Input: part model. Units: mm. Frame: model coordinates. Face numbers are marked on the shaded views. A direction names the side the tool comes from. Coordinates: 2 decimals unless noted, no trailing zeros. Write each loop counter-clockwise with the first axis right and the second up, starting at its lowest first coordinate (ties: lowest second). Pieces come first, ordered by that corner, then holes. Notation, with made-up numbers: (66, 16) - (118, 16) arc R34 ccw to (118, 55) - close; hole circle Ø3 at (85, 67.25). An arc over 180 degrees is marked (long way). Use a Markdown table: item, result. Add a question column.
Q1. Pin query (flat end, axial travel): P1, Ø8, axis at x = 9, y = -29, coming from the -Z side; P2, Ø3.5, axis at y = -22.225, z = 0, coming from the +X side; P3, Ø1, axis at x = 15.5, z = -0.5, coming from the +Y side; P4, Ø12, axis at y = -14.5, z = -1, coming from the +X side. Return the tip coordinate at first contact, or that it passes through.
Q2. Section query D-D (z = 0). Give the number of separate pieces and of enclosed holes in the cut face, then the cut area to 3 significant figures.
Q3. Section query A-A (z = -5.25). Return the cut outline in (x, y).
Q4. Section query B-B (y = -17). Return the cut outline in (x, z), then the cut area to 3 significant figures.
Q5. Section query C-C (x = 13.5). Return the cut outline in (y, z).
Q6. Set-up query: the marked faces 1 and 2. Return all of +Z, -Z, +X, -X, +Y, -Y with unobstructed straight access to the full face (end or side cutting, diameter ignored); none if empty.
Q7. Material intervals for probe 1 along Y at (x, z) = (0.55, 0); probe 2 along Y at (x, z) = (-0.3, 0); probe 3 along X at (y, z) = (-19.5, 10), sorted ascending. Write a range as from..to.
from build123d import *

# Parameters (mm, degrees)
SKETCH2_W                       = 3.175
SKETCH2_H                       = 25.4
F_1_8_0_125_DIAMETER_HOLE1_D    = 3.175
F_3_32_0_09375_DIAMETER_HOLE2_D = 2.38125
FILLET1_R                       = 12.7
FILLET2_R                       = 6.35
CHAMFER3_SIZE                   = 0.762
CHAMFER2_SIZE                   = 0.254


with BuildPart() as part:
    # Sweep1: sweep along a path in Sketch1
    with BuildLine(Plane.XY) as sweep1_path:
        Line((0, 0), (0, -31.75))
        Line((0, -31.75), (0, -70.0334134))
        Line((0, -70.0334134), (27.49630657, -85.9084134))
    # Sketch2 → Sweep1 (sweep)
    with BuildSketch(Plane(origin=(0, 0, 0), x_dir=(1, 0, 0), z_dir=(0, 1, 0))):
        Rectangle(SKETCH2_W, SKETCH2_H)
    sweep(path=sweep1_path.line, transition=Transition.RIGHT)

    # 1/8 (0.125) Diameter Hole1 (through all)
    with Locations(Plane(origin=(1.5875, 0, 0), x_dir=(0, 0, -1), z_dir=(1, 0, 0))):
        with Locations((0, -9.525), (0, -22.225)):
            Hole(F_1_8_0_125_DIAMETER_HOLE1_D / 2)

    # 3/32 (0.09375) Diameter Hole2 (through all)
    with Locations(Plane(origin=(-29.531607559, -51.150244721, 0), x_dir=(0.866025404, -0.5, 0), z_dir=(0.5, 0.866025404, 0))):
        with Locations((57.2417067, 0)):
            Hole(F_3_32_0_09375_DIAMETER_HOLE2_D / 2)

    # Fillet1
    fillet1_edges = [part.edges().sort_by_distance(p)[0] for p in [
        (1.5875, -69.116869848, 0),
        (-1.5875, -70.949956952, 0),
    ]]
    fillet(fillet1_edges, radius=FILLET1_R)

    # Fillet2
    fillet2_edges = [part.edges().sort_by_distance(p)[0] for p in [
        (27.49630657, -85.9084134, -12.7),
        (27.49630657, -85.9084134, 12.7),
        (0, 0, -12.7),
        (0, 0, 12.7),
    ]]
    fillet(fillet2_edges, radius=FILLET2_R)

    # Chamfer3
    chamfer3_edges = [part.edges().sort_by_distance(p)[0] for p in [
        (12.982897628, -79.362179945, -12.7),
        (12.982897628, -79.362179945, 12.7),
        (15.364147628, -77.070821064, -12.7),
        (0.113977372, -69.967608534, -12.7),
        (0.113977372, -69.967608534, -12.7),
        (0.113977372, -69.967608534, 12.7),
        (15.364147628, -77.070821064, 12.7),
        (0.113977372, -69.967608534, 12.7),
        (3.288977372, -68.134521429, 12.7),
        (3.288977372, -68.134521429, 12.7),
        (3.288977372, -68.134521429, -12.7),
        (3.288977372, -68.134521429, -12.7),
        (1.5875, -34.067260714, 12.7),
        (1.5875, -34.067260714, -12.7),
        (-1.5875, -34.983804267, -12.7),
        (-1.5875, -34.983804267, 12.7),
        (26.70255657, -87.283228729, 0),
        (25.091860223, -86.353292759, 10.840128061),
        (25.091860223, -86.353292759, -10.840128061),
        (28.29005657, -84.533598071, 0),
        (26.679360223, -83.603662102, 10.840128061),
        (26.679360223, -83.603662102, -10.840128061),
        (1.5875, 0, 0),
        (-1.5875, 0, 0),
        (-1.5875, -34.983804267, 12.7),
        (-1.5875, -34.983804267, -12.7),
        (-1.5875, -1.859871939, 10.840128061),
        (-1.5875, -1.859871939, -10.840128061),
        (1.5875, -34.067260714, -12.7),
        (1.5875, -34.067260714, 12.7),
        (1.5875, -1.859871939, 10.840128061),
        (1.5875, -1.859871939, -10.840128061),
    ]]
    chamfer(chamfer3_edges, length=CHAMFER3_SIZE)

    # Chamfer2
    chamfer2_edges = [part.edges().sort_by_distance(p)[0] for p in [
        (1.5875, -22.225, -1.5875),
        (-1.5875, -22.225, -1.5875),
        (1.5875, -9.525, -1.5875),
        (-1.5875, -9.525, -1.5875),
        (19.484776095, -83.116041229, 0),
        (21.072276095, -80.366410571, 0),
    ]]
    chamfer(chamfer2_edges, length=CHAMFER2_SIZE)


solid = part.part
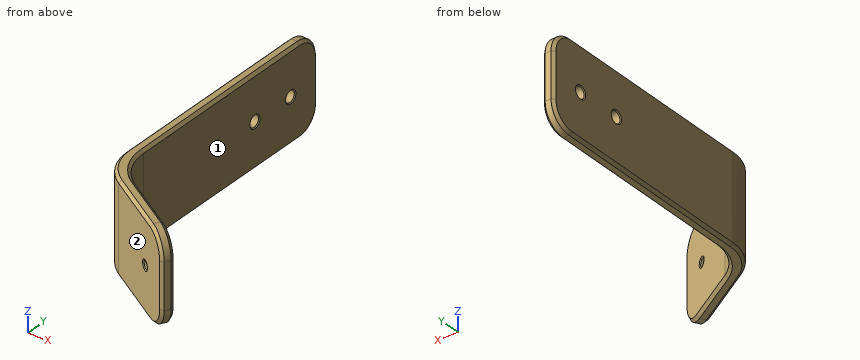
Values follow:
| question | item | result |
|---|---|---|
| 1 | P1 | through |
| 1 | P2 | x = 1.5 |
| 1 | P3 | y = -76.86 |
| 1 | P4 | x = 1.59 |
| 2 | separate pieces | 4 |
| 2 | enclosed holes | 0 |
| 2 | area | 294 mm2 |
| 3 | outline | (-1.59, -63.62) arc R12.7 ccw to (4.76, -74.62) - (26.04, -86.9) - (27.08, -86.62) - (27.91, -85.19) - (27.63, -84.15) - (7.94, -72.78) arc R12.7 cw to (1.59, -61.78) - (1.59, -0.76) - (0.83, 0) - (-0.83, 0) - (-1.59, -0.76) - close |
| 4 | outline | (-1.59, -11.94) - (-0.83, -12.7) - (0.83, -12.7) - (1.59, -11.94) - (1.59, 11.94) - (0.83, 12.7) - (-0.83, 12.7) - (-1.59, 11.94) - close |
| 4 | area | 79.5 mm2 |
| 5 | outline | (-79.66, -11.94) - (-78.78, -12.7) - (-76.87, -12.7) - (-75.99, -11.94) - (-75.99, 11.94) - (-76.87, 12.7) - (-78.78, 12.7) - (-79.66, 11.94) - close |
| 6 | face 1 | +Z, -Z, +X, +Y |
| 6 | face 2 | +Z, -Z, -X, -Y |
| 7 | probe 1 | -70.67..-23.81, -20.64..-11.11, -7.94..0 |
| 7 | probe 2 | -69.19..-23.81, -20.64..-11.11, -7.94..0 |
| 7 | probe 3 | -1.59..1.59 |
